from build123d import *

# Parameters (mm, degrees)
PAD004_DEPTH           = 20
SKETCH013_R            = 2.6
POCKET008_DEPTH        = 100
POCKET009_DEPTH        = 40
PAD005_DEPTH           = 70.3
SKETCH016_R            = 2.6
POCKET010_DEPTH        = 10
SKETCH017_R            = 2.6
POCKET011_DEPTH        = 10
SKETCH018_W            = 10
SKETCH018_H            = 1
POCKET012_DEPTH        = 25
SKETCH019_W            = 16.8
SKETCH019_H            = 21
PAD006_DEPTH           = 5.8
SKETCH020_W            = 12.8
SKETCH020_H            = 6
POCKET013_DEPTH        = 5.8
SKETCH021_W            = 16.8
SKETCH021_H            = 2
PAD007_DEPTH           = 1
SKETCH022_R            = 2
POCKET014_DEPTH        = 40
LINEARPATTERN001_COUNT = 3
LINEARPATTERN001_PITCH = 6
SKETCH023_R            = 1.6
POCKET015_DEPTH        = 12


with BuildPart() as part:
    # Sketch012 → Pad004 (new body)
    with BuildSketch(Plane.XZ):
        Polygon((17.1, 10.100008), (17.1, -4.899992), (25.3, -13.099992), (35.3, -13.099992), (35.3, -20.099992), (-35.3, -20.099992), (-35.3, -13.099992), (-25.3, -13.099992), (-17.1, -4.899992), (-17.1, 10.100008), (-17.1, 20.100008), (17.1, 20.100008), align=None)
        Polygon((-10.1, 10.100008), (-10.1, 4.900008), (-8.3, 3.099992), (-8.3, -3.100008), (-10.1, -4.899992), (-10.1, -10.099992), (-5.478931, -10.099992), (-5.478931, -11.099992), (5.478931, -11.099992), (5.478931, -10.099992), (10.1, -10.099992), (10.1, -4.899992), (8.3, -3.099992), (8.3, 3.100008), (10.1, 4.900008), (10.1, 10.100008), align=None, mode=Mode.SUBTRACT)
    extrude(amount=PAD004_DEPTH)

    # Sketch013 (on Face22 of Pad004) → Pocket008 (cut)
    with BuildSketch(Plane(origin=(8.3, 0, 0), x_dir=(0, 0, -1), z_dir=(-1, 0, 0))):
        with Locations((0, 10)):
            Circle(SKETCH013_R)
    extrude(amount=-POCKET008_DEPTH, mode=Mode.SUBTRACT)

    # Sketch013 (on Face22 of Pad004) → Pocket009 (cut)
    with BuildSketch(Plane(origin=(8.3, 0, 0), x_dir=(0, 0, -1), z_dir=(-1, 0, 0))):
        with Locations((0, 10)):
            Circle(SKETCH013_R)
    extrude(amount=POCKET009_DEPTH, mode=Mode.SUBTRACT)

    # Sketch015 → Pad005 (join)
    with BuildSketch(Plane(origin=(35.15, 0, 0), x_dir=(0, 0, 1), z_dir=(1, 0, 0))):
        Polygon((-20.000008, 14.8), (-20.000008, 5), (-21.800008, 6.8), (-21.800008, 13), align=None)
    extrude(amount=-PAD005_DEPTH)

    # Sketch016 (on Face3 of Pad005) → Pocket010 (cut)
    with BuildSketch(Plane(origin=(0, 0, -13.099992), x_dir=(-1, 0, 0), z_dir=(0, 0, 1))):
        with Locations((-30.3, 10)):
            Circle(SKETCH016_R)
    extrude(amount=-POCKET010_DEPTH, mode=Mode.SUBTRACT)

    # Sketch017 (on Face12 of Pocket010) → Pocket011 (cut)
    with BuildSketch(Plane(origin=(0, 0, -13.099992), x_dir=(-1, 0, 0), z_dir=(0, 0, 1))):
        with Locations((30.3, 10)):
            Circle(SKETCH017_R)
    extrude(amount=-POCKET011_DEPTH, mode=Mode.SUBTRACT)

    # Sketch018 (on Face4 of Pocket011) → Pocket012 (cut)
    with BuildSketch(Plane(origin=(0, 0, 0), x_dir=(1, 0, 0), z_dir=(0, 1, 0))):
        with Locations((0.1, -10.600008)):
            Rectangle(SKETCH018_W, SKETCH018_H)
    extrude(amount=-POCKET012_DEPTH, mode=Mode.SUBTRACT)

    # Sketch019 (on Face6 of Pocket012) → Pad006 (join)
    with BuildSketch(Plane(origin=(0, 0, 20.100008), x_dir=(-1, 0, 0), z_dir=(0, 0, 1))):
        with Locations((0, 9.5)):
            Rectangle(SKETCH019_W, SKETCH019_H)
    extrude(amount=PAD006_DEPTH)

    # Sketch020 (on Face46 of Pad006) → Pocket013 (cut)
    with BuildSketch(Plane(origin=(0, 0, 25.900008), x_dir=(-1, 0, 0), z_dir=(0, 0, 1))):
        with Locations((0, 2)):
            Rectangle(SKETCH020_W, SKETCH020_H)
    extrude(amount=-POCKET013_DEPTH, mode=Mode.SUBTRACT)

    # Sketch021 (on Face4 of Pocket013) → Pad007 (join)
    with BuildSketch(Plane(origin=(0, 0, 0), x_dir=(1, 0, 0), z_dir=(0, 1, 0))):
        with Locations((0, -19.100008)):
            Rectangle(SKETCH021_W, SKETCH021_H)
    extrude(amount=PAD007_DEPTH)

    # Sketch022 (on Face46 of Pad007) → Pocket014 (cut)
    with BuildSketch(Plane(origin=(0, -5, 0), x_dir=(1, 0, 0), z_dir=(0, 1, 0))):
        with Locations((-6.4, -23.000008)):
            Circle(SKETCH022_R)
    pocket014 = extrude(amount=-POCKET014_DEPTH, mode=Mode.SUBTRACT)

    # LinearPattern001: Pocket014 ×3
    with Locations(*[(i * LINEARPATTERN001_PITCH, 0, 0) for i in range(1, LINEARPATTERN001_COUNT)]):
        add(pocket014, mode=Mode.SUBTRACT)

    # Sketch023 (on Face5 of LinearPattern001) → Pocket015 (cut)
    with BuildSketch(Plane.XZ.offset(20)):
        with Locations((0, 16.970566)):
            Circle(SKETCH023_R)
    extrude(amount=-POCKET015_DEPTH, mode=Mode.SUBTRACT)


solid = part.part
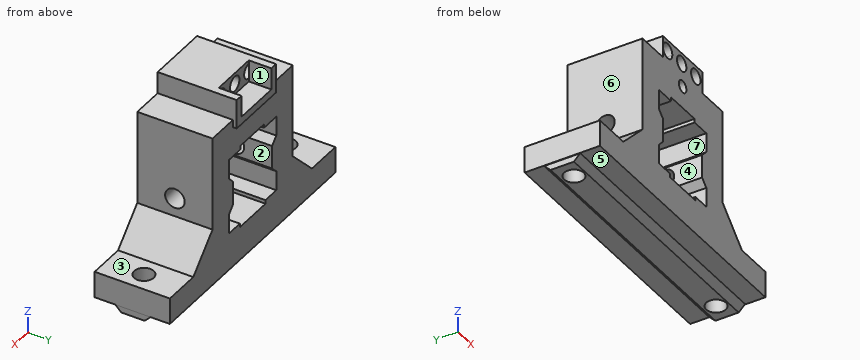
For this review, take the finished solid that the model builds, in its own axes (mm). Face numbers are marked on the shaded views. A direction names the side the tool comes from. Give positions to 0.01 mm unless a question says otherwise; leave off trailing zeros. Order: outer loops, then holes, each group sorted by start corner. A loop starts at its lowest first (then second) coordinate and runs counter-clockwise, first axis right, second up. Notation, with made-up numbers: M 59,28 L 112,28 A27 cw 112,46 Z; hole C -25,64 d5. An arc over 180 degrees is marked long. Answer in a Markdown table with one row per item. Add a question column.
(1) Mouldability with a two-part tool opening along Z and no side actions: class the marked faces 4, 5, 6 and 7 as +Z half, -Z half, draft (parallel to the pull), parting line (faces both ways), or undercut.
(2) Consider section A-A on z = -7.5. State the section outline as (x, y) points.
(3) For the marked faces 1, 2 and 3, list the 3-axis set-ups (+Z, -Z, +X, -X, +Y, -Y) from which the entire face can be reached by the end or side of a thin tool; tool diameter is ignored.
(4) Wall thickness on probe 1 along X at (y, z) = (-10, -20); probe 2 along Z at (x, y) = (13, -10); probe 3 along X at (y, z) = (-9.5, 9): over which ranges is each line inside the solid? List them lowest first. Write a range as [from, to].
(5) Consider section B-B on x = 30.3. State the section outline as (y, z) points.
(6) Consider section D-D on x = 20.5. State the section outline as (y, z) points.
(7) For pin 1 (1.5 mm diameter, centred on x = -4, y = -5.5, fed in from -Z); pin 2 (0.5 mm diameter, centred on x = -2, y = 0.5, fed in from -Z); pin 3 (12 mm diameter, centred on x = 21.5, y = -2, fed in from -Z); pin 4 (2.5 mm diameter, centred on y = -8.5, z = 21, fed in from +X), all flat-tipped, find the tip position at first contact; note any pin that passes through.
(8) Consider section C-C on z = 0. State the section outline as (x, y) points.
Evaluation:
| question | item | result |
|---|---|---|
| 1 | face 4 | undercut |
| 1 | face 5 | -Z half |
| 1 | face 6 | draft |
| 1 | face 7 | undercut |
| 2 | outline | M -19.7,-20 L -10.1,-20 L -10.1,0 L -19.7,0 Z; M 10.1,-20 L 19.7,-20 L 19.7,0 L 10.1,0 Z |
| 3 | face 1 | +Z, +Y |
| 3 | face 2 | +Y, -Y |
| 3 | face 3 | +Z, +X, +Y, -Y |
| 4 | probe 1 | x = [-35.3, -32.9], [-27.7, 27.7], [32.9, 35.3] |
| 4 | probe 2 | z = [-21.8, -2.6], [2.6, 20.1] |
| 4 | probe 3 | x = [-17.1, -10.1], [10.1, 17.1] |
| 5 | outline | M -20,-20.1 L -14.7,-20.1 L -13,-21.8 L -12.6,-21.8 L -12.6,-13.1 L -20,-13.1 Z; M -7.4,-21.8 L -6.8,-21.8 L -5.1,-20.1 L 0,-20.1 L 0,-13.1 L -7.4,-13.1 Z |
| 6 | outline | M -20,-20.1 L -14.7,-20.1 L -13,-21.8 L -6.8,-21.8 L -5.1,-20.1 L 0,-20.1 L 0,-8.3 L -20,-8.3 Z |
| 7 | pin 1 | stops at z = -21.25 |
| 7 | pin 2 | stops at z = 18.1 |
| 7 | pin 3 | stops at z = -21.8 |
| 7 | pin 4 | stops at x = 17.1 |
| 8 | outline | M -17.1,-20 L -8.3,-20 L -8.3,-12.6 L -17.1,-12.6 Z; M -17.1,-7.4 L -8.3,-7.4 L -8.3,0 L -17.1,0 Z; M 8.3,-20 L 17.1,-20 L 17.1,-12.6 L 8.3,-12.6 Z; M 8.3,-7.4 L 17.1,-7.4 L 17.1,0 L 8.3,0 Z |
